```python
from build123d import *

# Parameters (mm, degrees)
F0_W     = 6.35
F0_H     = 12.7
F0_H_2   = 6.35
F0_W_2   = 69.85
F1_DEPTH = 25.4
F2_DEPTH = 25.4


with BuildPart() as f1:
    # F0 (on Front) → F1 (new body)
    with BuildSketch(Plane.XZ):
        with Locations((-34.925, 0)):
            Rectangle(F0_W, F0_H)
        with Locations((-34.925, 9.525)):
            Rectangle(F0_W, F0_H_2)
        with Locations((3.175, 0)):
            Rectangle(F0_W_2, F0_H)
    extrude(amount=F1_DEPTH)

    # F0 (on Front) + F1_face (on face) → F2 (join)
    with BuildSketch(Plane.XZ):
        with Locations((-34.925, 9.525)):
            Rectangle(F0_W, F0_H_2)
        with Locations((-34.925, 0)):
            Rectangle(F0_W, F0_H)
        with Locations((3.175, 0)):
            Rectangle(F0_W_2, F0_H)
    with BuildSketch(Plane(origin=(-1.397, -25.4, 0.381), x_dir=(1, 0, 0), z_dir=(0, -1, 0))):
        Polygon((-36.703, 12.319), (-36.703, -6.731), (39.497, -6.731), (39.497, 5.969), (-30.353, 5.969), (-30.353, 12.319), align=None)
    extrude(amount=F2_DEPTH)


solid = f1.part
```
Can you work these out from the model? Positions are in its coordinate system, mm. Round coordinates to 2 decimals unless told otherwise and drop trailing zeros. Loops run counter-clockwise (first coordinate to the right, second up) from the corner with the lowest first, then second, coordinate; pieces in that order, holes last. Notation, with made-up numbers: (-19, 27.5) -> (28, 27.5) arc R22 cw to (28, 34.5) -> close; hole circle Ø9 at (2.5, -20.75). An arc over 180 degrees is marked (long way). Answer in a Markdown table with one row per item.
Item 1: Suppose I cut it at C-C, the plane z = 10.25. List the corners of the cut face in (x, y) for me, plus the area to 3 significant figures.
Answer block:
| item | result |
|---|---|
| outline | (-38.1, -50.8) -> (-31.75, -50.8) -> (-31.75, 0) -> (-38.1, 0) -> close |
| area | 323 mm² |
Item 2: Suppose I cut it at B-B, the plane x = 16.5. List the corners of the cut face in (y, z) for me, plus the area to 3 significant figures.
Answer block:
| item | result |
|---|---|
| outline | (-50.8, -6.35) -> (0, -6.35) -> (0, 6.35) -> (-50.8, 6.35) -> close |
| area | 645 mm² |
Item 3: We'd pull the mould along Z, two halves only. Please class faces 1 (the flat face through (3, -25, 6.35)), 2 (the flat face through (-31.75, -25, 9)), 3 (the flat face through (-1, -25, -6.35)): released by +Z, released by -Z, zero draft, split by the parting line, or undercut.
Answer block:
| item | result |
|---|---|
| face 1 | released by +Z |
| face 2 | zero draft |
| face 3 | released by -Z |
Item 4: If I drill on probe 1 along Z at (x, y) = (35, -15.5); probe 2 along X at (y, z) = (-29, 8.25), over which ranges is the centre line in solid material (lowest first)?
Answer block:
| item | result |
|---|---|
| probe 1 | -6.35 to 6.35 |
| probe 2 | -38.1 to -31.75 |
Item 5: Suppose I cut it at A-A, the plane y = -30. List the corners of the cut face in (x, z) for me, plus the area to 3 significant figures.
Answer block:
| item | result |
|---|---|
| outline | (-38.1, -6.35) -> (38.1, -6.35) -> (38.1, 6.35) -> (-31.75, 6.35) -> (-31.75, 12.7) -> (-38.1, 12.7) -> close |
| area | 1,010 mm² |
Item 6: Will this pin go through, and if not, where does the flat tip stop? P1, Ø3, axis at y = -22.5, z = 10, coming from the +X side.
Answer block:
| item | result |
|---|---|
| P1 | x = -31.75 |
